Model file for the job. Use its own axes, mm. A direction names the side the tool comes from. Give positions to 0.01 mm unless a question says otherwise; leave off trailing zeros. Write each loop counter-clockwise with the first axis right and the second up, starting at its lowest first coordinate (ties: lowest second). Pieces come first, ordered by that corner, then holes.
```python
from build123d import *

# Parameters (mm, degrees)
SKETCH1_W              = 133.35
SKETCH1_H              = 120.65
BOSS_EXTRUDE1_DEPTH    = 3.175
SKETCHED_START         = -120.65
SKETCHED_BEND1_DEPTH   = 120.65
SKETCHED_BEND1_2_DEPTH = 120.65
CUT_EXTRUDE1_DEPTH     = 157.911861269
SKETCH9_R              = 1.5875
CUT_EXTRUDE2_DEPTH     = 158.831464015
FILLET1_R              = 3.175


# Read off the part's stored shape, not the designer's step: Sketched Bend1
with BuildPart() as part:
    # Sketch1 → Boss-Extrude1 (new body)
    with BuildSketch(Plane(origin=(0, 0, 0), x_dir=(1, 0, 0), z_dir=(0, 1, 0))):
        with Locations((66.675, 60.325)):
            Rectangle(SKETCH1_W, SKETCH1_H)
    extrude(amount=BOSS_EXTRUDE1_DEPTH)

    # Sketched Bend1 outline → Sketched Bend1 (cut)
    with BuildSketch(Plane.XY.offset(SKETCHED_START)):
        with BuildLine():
            Line((133.35, 3.175), (91.224261315, 3.175))
            ThreePointArc((91.224261315, 3.175), (88.900000001, 0.850738686), (85.725, 0))
            Line((85.725, 0), (133.35, 0))
            Line((133.35, 0), (133.35, 3.175))
        make_face()
    extrude(amount=SKETCHED_BEND1_DEPTH, mode=Mode.SUBTRACT)

    # Sketched Bend1 2 outline → Sketched Bend1 2 (add)
    with BuildSketch(Plane.XY.offset(SKETCHED_START)):
        with BuildLine():
            Line((88.9, 46.494082494), (88.9, 6.35))
            ThreePointArc((88.9, 6.35), (87.97006403, 4.10493597), (85.725, 3.175))
            Line((85.725, 3.175), (91.224261315, 3.175))
            ThreePointArc((91.224261315, 3.175), (91.858628997, 4.706499064), (92.075, 6.35))
            Line((92.075, 6.35), (92.075, 46.494082494))
            Line((92.075, 46.494082494), (88.9, 46.494082494))
        make_face()
    extrude(amount=SKETCHED_BEND1_2_DEPTH)

    # Sketch7 → Cut-Extrude1 (cut, through all)
    with BuildSketch(Plane.ZY.offset(-88.9)):
        with BuildLine():
            Line((-79.375, 46.494082494), (-79.375, 40.144082494))
            ThreePointArc((-79.375, 40.144082494), (-60.325, 21.094082494), (-41.275, 40.144082494))
            Line((-41.275, 40.144082494), (-41.275, 46.494082494))
            Line((-41.275, 46.494082494), (-79.375, 46.494082494))
        make_face()
    extrude(amount=-CUT_EXTRUDE1_DEPTH, mode=Mode.SUBTRACT)

    # Sketch9 → Cut-Extrude2 (cut, through all)
    with BuildSketch(Plane(origin=(0, 3.175, 0), x_dir=(1, 0, 0), z_dir=(0, 1, 0))):
        with Locations(Location((6.35, 114.3, 0), (0, 0, 270))):
            Circle(SKETCH9_R)
        with Locations(Location((79.375, 114.3, 0), (0, 0, 270))):
            Circle(SKETCH9_R)
        with Locations(Location((6.35, 6.35, 0), (0, 0, 270))):
            Circle(SKETCH9_R)
        with Locations(Location((79.375, 6.35, 0), (0, 0, 270))):
            Circle(SKETCH9_R)
    extrude(amount=-CUT_EXTRUDE2_DEPTH, mode=Mode.SUBTRACT)

    # Fillet1
    fillet1_edges = [part.edges().sort_by_distance(p)[0] for p in [
        (0, 1.5875, 0),
        (0, 1.5875, -120.65),
        (90.4875, 46.494082494, -79.375),
        (90.4875, 46.494082494, -41.275),
        (90.4875, 46.494082494, -120.65),
        (90.4875, 46.494082494, 0),
    ]]
    fillet(fillet1_edges, radius=FILLET1_R)


solid = part.part
```
1. Slice it at D-D, the plane z = -71.5. Write the cut outline in (x, y) (3 decimals).
Calculated:
outline: (0, 0) - (85.725, 0) arc R6.35 ccw to (92.075, 6.35) - (92.075, 24.716) - (88.9, 24.716) - (88.9, 6.35) arc R3.175 cw to (85.725, 3.175) - (0, 3.175) - close
2. Which spindle directions (+Z, -Z, +X, -X, +Y, -Y) get a long thin tool onto all of the face, cutting with end or side? Do faces 4 (the flat face through (88.9, 18, -61)), 5 (the flat face through (90, 42, -41.275)), 6 (the flat face through (61, 3, 0)). Say none if no direction does.
Calculated:
face 4: +Z, -Z, -X, +Y
face 5: +X, -X, +Y
face 6: +Z, +X, -X, +Y, -Y
3. Slice it at C-C, the plane y = 37. Write the cut outline in (x, z) (3 decimals), and give its area (3 significant figures).
Calculated:
outline: (88.9, -120.65) - (92.075, -120.65) - (92.075, -79.114) - (88.9, -79.114) - close; (88.9, -41.536) - (92.075, -41.536) - (92.075, 0) - (88.9, 0) - close
area: 264 mm2
4. Slice it at A-A, the plane z = -6.35. State how many separate pieces and enclosed holes the cut face has, and give its area (3 significant figures).
Calculated:
separate pieces: 3
enclosed holes: 0
area: 403 mm2
5. Pin check, flat tip, straight feed: P1, Ø3, axis at x = 12, z = -18.5, coming from the +Y side (3 decimals). Stop position of the tip, or through.
Calculated:
P1: stops at y = 3.175
6. Pull direction X, two halves, no side cores. Call faces 1 (the cylindrical face through (80.45, 1.61, -115.47)), 2 (the cylindrical face through (0.95, 1.61, -0.91)), 3 (the flat face through (42, 0, -61)): +X half, -X half, draft (parallel to the pull), parting line (faces both ways), or undercut.
Calculated:
face 1: undercut
face 2: -X half
face 3: draft
7. Probe probe 1 along X at (y, z) = (1, -114); probe 2 along Y at (x, z) = (25.5, -62) (3 decimals); probe 3 along X at (y, z) = (1.9, -114.3). List the from-to ranges inside material, lowest first.
Calculated:
probe 1: x = 0 to 4.79, 7.91 to 77.82, 80.93 to 89.15
probe 2: y = 0 to 3.175
probe 3: x = 0 to 4.76, 7.94 to 77.79, 80.96 to 90.25
